Read the model definition and answer for the solid it produces. Units are mm, in the model's axes. Face numbers are marked on the shaded views. A direction names the side the tool comes from. Round coordinates to 2 decimals unless told otherwise and drop trailing zeros. Write each loop counter-clockwise with the first axis right and the second up, starting at its lowest first coordinate (ties: lowest second). Pieces come first, ordered by that corner, then holes. Notation, with made-up numbers: (10, -9.75) - (54, -9.75) arc R17 ccw to (54, 14.25) - close; hole circle Ø1 at (23.5, -19.5). An arc over 180 degrees is marked (long way). Use one line per item in the form item = value. Start each with the question number.
1) For a pull along Z with two mould halves and no side action, classify the marked faces 4, 5, 6 and 7 as released by +Z, released by -Z, zero draft, split by the parting line, or undercut.
2) The part is cut by section C-C, the plane z = -1. Give the vertices of the cut face in (x, y), plus the area to 3 significant figures.
3) The part is cut by section D-D, the plane y = -15. Give the vertices of the cut face in (x, z).
4) The part is cut by section A-A, the plane y = -20.5. Give the vertices of the cut face in (x, z).
5) Consider line 1 along X through (y, z) = (-13, 6); line 2 along Z through (x, y) = (21, -17); line 3 along Y through (x, z) = (33, 13.5). Determine where each line is inside the solid, lowest interval first. Write a range as from..to.
6) Each of these flat-tipped pins is pushed along its axis until it touches: pin 1 (6.5 mm diameter, centred on x = 7, z = -15, fed in from -Y); pin 2 (14.5 mm diameter, centred on y = -13.13, z = 13.13, fed in from +X). Where does it stop, or does it pass through?
7) For the marked faces 1, 2 and 3, determine the directions among +Z, -Z, +X, -X, +Y, -Y from which every point of the face is accessible in a straight line to the end or side of a thin tool.
8) The part is cut by section B-B, the plane x = 23.5. Give the vertices of the cut face in (y, z), plus the area to 3 significant figures.
from build123d import *

# Parameters (mm, degrees)
F0_W     = 63.3814185858
F0_H     = 8.4347892553
F1_DEPTH = 25.4
F2_W     = 44.3428922445
F2_H     = 12.5068214998
F3_DEPTH = 100.838
F4_R     = 5.5480982764
F5_DEPTH = 130.048


with BuildPart() as f1:
    # F0 (on Front) → F1 (new body)
    with BuildSketch(Plane.XZ):
        with Locations((-4.3378919363, -13.736656867)):
            Rectangle(F0_W, F0_H)
        Polygon((-36.0286012292, -17.9540514946), (-36.0286012292, -9.5192622393), (-36.0286012292, 32.654684037), (-44.7043813765, 32.654684037), (-44.7043813765, -17.9540514946), align=None)
        Polygon((27.3528173566, 32.654684037), (27.3528173566, -9.5192622393), (27.3528173566, -17.9540514946), (36.9925759733, -17.9540514946), (36.9925759733, 44.4633886218), (27.3528173566, 44.4633886218), align=None)
        Polygon((-44.7043813765, 32.654684037), (-36.0286012292, 32.654684037), (27.3528173566, 32.654684037), (27.3528173566, 44.4633886218), (-44.7043813765, 44.4633886218), align=None)
    extrude(amount=F1_DEPTH)

    # F2 (on face) → F3 (cut)
    with BuildSketch(Plane(origin=(0, 0, -17.9540514946), x_dir=(1, 0, 0), z_dir=(0, 0, -1))):
        with Locations((-1.5664612874, 19.1465892501)):
            Rectangle(F2_W, F2_H)
    extrude(amount=-F3_DEPTH, mode=Mode.SUBTRACT)

    # F4 (on face) → F5 (cut)
    with BuildSketch(Plane.YZ.offset(36.9925759733)):
        with Locations((-13.1341712549, 13.1341721863)):
            Circle(F4_R)
    extrude(amount=-F5_DEPTH, mode=Mode.SUBTRACT)


solid = f1.part
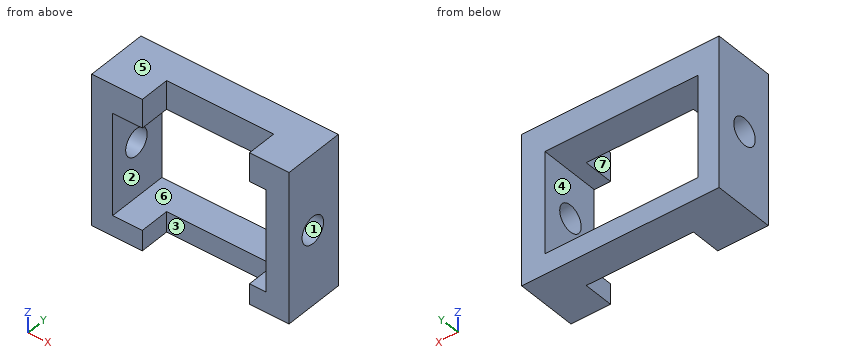
Geometry results:
q1.face_4 = undercut
q1.face_5 = released by +Z
q1.face_6 = undercut
q1.face_7 = zero draft
q2.outline = (-44.7, -25.4) - (-36.03, -25.4) - (-36.03, 0) - (-44.7, 0) - close; (27.35, -25.4) - (36.99, -25.4) - (36.99, 0) - (27.35, 0) - close
q2.area = 465 mm2
q3.outline = (-44.7, -17.95) - (-23.74, -17.95) - (-23.74, -9.52) - (-36.03, -9.52) - (-36.03, 7.91) - (-44.7, 7.91) - close; (-44.7, 18.36) - (-36.03, 18.36) - (-36.03, 32.65) - (-23.74, 32.65) - (-23.74, 44.46) - (-44.7, 44.46) - close; (20.6, -17.95) - (36.99, -17.95) - (36.99, 7.91) - (27.35, 7.91) - (27.35, -9.52) - (20.6, -9.52) - close; (20.6, 32.65) - (27.35, 32.65) - (27.35, 18.36) - (36.99, 18.36) - (36.99, 44.46) - (20.6, 44.46) - close
q4.outline = (-44.7, -17.95) - (-23.74, -17.95) - (-23.74, -9.52) - (-36.03, -9.52) - (-36.03, 32.65) - (-23.74, 32.65) - (-23.74, 44.46) - (-44.7, 44.46) - close; (20.6, -17.95) - (36.99, -17.95) - (36.99, 44.46) - (20.6, 44.46) - (20.6, 32.65) - (27.35, 32.65) - (27.35, -9.52) - (20.6, -9.52) - close
q5.line_1 = -44.7..-36.03, 27.35..36.99
q5.line_2 = -17.95..-9.52, 32.65..44.46
q5.line_3 = -25.4..-18.67, -7.6..0
q6.pin_1 = -12.89
q6.pin_2 = 36.99
q7.face_1 = +X, -X
q7.face_2 = +Y, -Y
q7.face_3 = +Z, -Z, -Y
q8.outline = (-25.4, -17.95) - (0, -17.95) - (0, -9.52) - (-25.4, -9.52) - close; (-25.4, 32.65) - (0, 32.65) - (0, 44.46) - (-25.4, 44.46) - close
q8.area = 514 mm2
